```python
from build123d import *

# Parameters (mm, degrees)
SKETCH1_R                               = 3
BOSS_EXTRUDE1_DEPTH                     = 18.75
SKETCH2_R                               = 5
CUT_EXTRUDE3_DEPTH                      = 5.5
CBORE_FOR_M5_HEX_HEAD_BOLT1_D           = 6
CBORE_FOR_M5_HEX_HEAD_BOLT1_CBORE_D     = 11
CBORE_FOR_M5_HEX_HEAD_BOLT1_CBORE_DEPTH = 5.5
CUT_EXTRUDE4_DEPTH                      = 40
CUT_EXTRUDE5_DEPTH                      = 4


with BuildPart() as part:
    # Sketch1 → Boss-Extrude1 (new body)
    with BuildSketch(Plane.XY):
        Polygon((88.518625365, 66.433253323), (-88.518625365, 66.433253323), (-88.518625365, 46.433253323), (-88.518625365, -4.066746677), (-88.518625365, -154.066746677), (88.518625365, -154.066746677), (88.518625365, -4.066746677), (88.518625365, 46.433253323), align=None)
        with Locations((83.018625365, 39.183253323)):
            Circle(SKETCH1_R, mode=Mode.SUBTRACT)
        with Locations((51.018625365, 39.183253323)):
            Circle(SKETCH1_R, mode=Mode.SUBTRACT)
        with Locations((83.018625365, 3.183253323)):
            Circle(SKETCH1_R, mode=Mode.SUBTRACT)
        with Locations((51.018625365, 3.183253323)):
            Circle(SKETCH1_R, mode=Mode.SUBTRACT)
        with Locations((83.018625365, -86.016746677)):
            Circle(SKETCH1_R, mode=Mode.SUBTRACT)
        with Locations((51.018625365, -86.016746677)):
            Circle(SKETCH1_R, mode=Mode.SUBTRACT)
        with Locations((51.018625365, -122.016746677)):
            Circle(SKETCH1_R, mode=Mode.SUBTRACT)
        with Locations((83.018625365, -122.016746677)):
            Circle(SKETCH1_R, mode=Mode.SUBTRACT)
        with Locations(Location((-83.018625365, -122.016746677, 0), (0, 0, 180))):
            Circle(SKETCH1_R, mode=Mode.SUBTRACT)
        with Locations(Location((-51.018625365, -122.016746677, 0), (0, 0, 180))):
            Circle(SKETCH1_R, mode=Mode.SUBTRACT)
        with Locations(Location((-51.018625365, -86.016746677, 0), (0, 0, 180))):
            Circle(SKETCH1_R, mode=Mode.SUBTRACT)
        with Locations(Location((-83.018625365, -86.016746677, 0), (0, 0, 180))):
            Circle(SKETCH1_R, mode=Mode.SUBTRACT)
        with Locations(Location((-51.018625365, 3.183253323, 0), (0, 0, 180))):
            Circle(SKETCH1_R, mode=Mode.SUBTRACT)
        with Locations(Location((-83.018625365, 3.183253323, 0), (0, 0, 180))):
            Circle(SKETCH1_R, mode=Mode.SUBTRACT)
        with Locations(Location((-51.018625365, 39.183253323, 0), (0, 0, 180))):
            Circle(SKETCH1_R, mode=Mode.SUBTRACT)
        with Locations(Location((-83.018625365, 39.183253323, 0), (0, 0, 180))):
            Circle(SKETCH1_R, mode=Mode.SUBTRACT)
    extrude(amount=BOSS_EXTRUDE1_DEPTH)

    # Sketch2 → Cut-Extrude3 (cut)
    with BuildSketch(Plane.XY.offset(18.75)):
        with Locations((-51.018625365, 39.183253323)):
            Circle(SKETCH2_R)
        with Locations((-83.018625365, 39.183253323)):
            Circle(SKETCH2_R)
        with Locations((-83.018625365, 3.183253323)):
            Circle(SKETCH2_R)
        with Locations((51.018625365, 39.183253323)):
            Circle(SKETCH2_R)
        with Locations((83.018625365, 39.183253323)):
            Circle(SKETCH2_R)
        with Locations((83.018625365, 3.183253323)):
            Circle(SKETCH2_R)
        with Locations((51.018625365, 3.183253323)):
            Circle(SKETCH2_R)
        with Locations((-51.018625365, 3.183253323)):
            Circle(SKETCH2_R)
        with Locations((-83.018625365, -86.016746677)):
            Circle(SKETCH2_R)
        with Locations((-51.018625365, -86.016746677)):
            Circle(SKETCH2_R)
        with Locations((-51.018625365, -122.016746677)):
            Circle(SKETCH2_R)
        with Locations((-83.018625365, -122.016746677)):
            Circle(SKETCH2_R)
        with Locations((51.018625365, -122.016746677)):
            Circle(SKETCH2_R)
        with Locations((51.018625365, -86.016746677)):
            Circle(SKETCH2_R)
        with Locations((83.018625365, -86.016746677)):
            Circle(SKETCH2_R)
        with Locations((83.018625365, -122.016746677)):
            Circle(SKETCH2_R)
    extrude(amount=-CUT_EXTRUDE3_DEPTH, mode=Mode.SUBTRACT)

    # CBORE for M5 Hex Head Bolt1 (through all)
    with Locations(Plane.XY.offset(18.75)):
        with Locations((-20, -1), (20, -1), (-20, -25), (20, -25)):
            CounterBoreHole(CBORE_FOR_M5_HEX_HEAD_BOLT1_D / 2, CBORE_FOR_M5_HEX_HEAD_BOLT1_CBORE_D / 2, CBORE_FOR_M5_HEX_HEAD_BOLT1_CBORE_DEPTH)

    # Sketch7 → Cut-Extrude4 (cut)
    with BuildSketch(Plane(origin=(0, 66.433253323, 0), x_dir=(1, 0, 0), z_dir=(0, 1, 0))):
        Polygon((-14.828427125, -2), (-16.828427125, -2), (-16.828427125, 0), (16.828427125, 0), (16.828427125, -2), (14.828427125, -2), align=None)
    extrude(amount=-CUT_EXTRUDE4_DEPTH, mode=Mode.SUBTRACT)

    # Sketch8 → Cut-Extrude5 (cut)
    with BuildSketch(Plane(origin=(0, 0, 0), x_dir=(-1, 0, 0), z_dir=(0, 0, -1))):
        with BuildLine():
            Line((18.941074346, 17.528523034), (18.941074346, 6.471477064))
            ThreePointArc((18.941074346, 6.471477064), (18.154389929, 5.908425795), (17.361427351, 5.354251227))
            Line((17.361427351, 5.354251227), (-17.361427384, 5.354251227))
            ThreePointArc((-17.361427384, 5.354251227), (-18.154389934, 5.908425774), (-18.941074346, 6.471476988))
            Line((-18.941074346, 6.471476988), (-18.941074346, 17.528522958))
            ThreePointArc((-18.941074346, 17.528522958), (-18.154389929, 18.091574227), (-17.361427351, 18.645748796))
            Line((-17.361427351, 18.645748796), (17.361427384, 18.645748796))
            ThreePointArc((17.361427384, 18.645748796), (18.154389934, 18.091574248), (18.941074346, 17.528523034))
        make_face()
    extrude(amount=-CUT_EXTRUDE5_DEPTH, mode=Mode.SUBTRACT)


solid = part.part
```
Verification items for the finished model (mm, model axes). A direction names the side the tool comes from. Coordinates: 2 decimals unless noted, no trailing zeros. Loops run counter-clockwise (first coordinate to the right, second up) from the corner with the lowest first, then second, coordinate; pieces in that order, holes last. Notation, with made-up numbers: (59.25, 72.5) - (96.25, 72.5) arc R19 ccw to (96.25, 98.5) - close; hole circle Ø11 at (75.25, 0). An arc over 180 degrees is marked (long way). Put each result on its own line as item: value.
Item 1: Section check A-A (y = -25). Enter the section's corners in (x, z).
Conclusion:
outline: (-88.52, 0) - (-23, 0) - (-23, 13.25) - (-25.5, 13.25) - (-25.5, 18.75) - (-88.52, 18.75) - close; (-17, 0) - (17, 0) - (17, 13.25) - (14.5, 13.25) - (14.5, 18.75) - (-14.5, 18.75) - (-14.5, 13.25) - (-17, 13.25) - close; (23, 0) - (88.52, 0) - (88.52, 18.75) - (25.5, 18.75) - (25.5, 13.25) - (23, 13.25) - close
Item 2: Gauge pin test, flat ends, axial feed: pin 1 Ø9 at (x, y) = (83.02, 39.18) entering from +Z; pin 2 Ø3.5 at (x, y) = (-83.02, 3.18) entering from -Z; pin 3 Ø10 at (x, y) = (5, 43.5) entering from -Z. Record the tip position at first contact, or that the pin passes through.
Conclusion:
pin 1: stops at z = 13.25
pin 2: passes through
pin 3: stops at z = 2
Item 3: Scan lines: line 1 along Y through (x, z) = (20, 16.65); line 2 along Y through (x, z) = (51, 11); line 3 along Y through (x, z) = (-80, 17.75). Record each from-to range of solid material in increasing order.
Conclusion:
line 1: y = -154.07 to -30.5, -19.5 to -6.5, 4.5 to 66.43
line 2: y = -154.07 to -125.02, -119.02 to -89.02, -83.02 to 0.18, 6.18 to 36.18, 42.18 to 66.43
line 3: y = -154.07 to -126, -118.03 to -90, -82.03 to -0.8, 7.17 to 35.2, 43.17 to 66.43
Item 4: Set-up check for faces 1 (the face through (0, 12, 4)), 2 (the face through (22.4, -3.4, 13.25)), 3 (the face through (-80.808, -88.044, 6.532)): record each of +Z, -Z, +X, -X, +Y, -Y from which the full face is reachable in a straight line by a thin tool's end or side.
Conclusion:
face 1: -Z
face 2: +Z
face 3: +Z, -Z
Item 5: Draft check along X on faces 4 (the face through (80.638, -123.842, 6.532)), 5 (the face through (-1, -42, 0)). Enter one of: pulls with the +X half, pulls with the -X half, needs draft (parallel to the pull), parting line crosses it, or undercut.
Conclusion:
face 4: undercut
face 5: needs draft
